```python
from build123d import *

# Parameters (mm, degrees)
SKETCH1_R               = 72.5
SKETCH1_R_2             = 62.5
BOSS_EXTRUDE1_DEPTH     = 10
SKETCH2_W               = 25
SKETCH2_H               = 10
BOSS_EXTRUDE2_DEPTH     = 100
SKETCH3_W               = 145
SKETCH3_H               = 50
BOSS_EXTRUDE3_DEPTH     = 10
CUT_EXTRUDE1_START      = -10
SKETCH4_R               = 62.5
CUT_EXTRUDE1_DEPTH      = 10
SKETCH5_W               = 145
SKETCH5_H               = 12.5
BOSS_EXTRUDE4_DEPTH     = 50
CUT_EXTRUDE2_DEPTH      = 138.318061449
CUT_EXTRUDE2_DEPTH_BACK = 138.318061449
SKETCH6_R               = 1.75
CUT_EXTRUDE3_DEPTH      = 138.318061449
CUT_EXTRUDE3_DEPTH_BACK = 138.318061449
SKETCH7_W               = 2.5
SKETCH7_H               = 7.5
SKETCH8_W               = 145
SKETCH8_H               = 12.5
CUT_EXTRUDE4_DEPTH      = 50
SKETCH9_W               = 145
SKETCH9_H               = 10
CUT_EXTRUDE5_DEPTH      = 87.5
SKETCH11_W              = 12.5
SKETCH11_H              = 10
CUT_EXTRUDE7_DEPTH      = 15
SKETCH13_W              = 12.5
SKETCH13_H              = 10
CUT_EXTRUDE9_DEPTH      = 50
SKETCH14_W              = 12.5
SKETCH14_H              = 10
CUT_EXTRUDE10_DEPTH     = 25


with BuildPart() as part:
    # Sketch1 → Boss-Extrude1 (new body)
    with BuildSketch(Plane(origin=(0, 0, 0), x_dir=(1, 0, 0), z_dir=(0, 1, 0))):
        with Locations(Location((0, 0, 0), (0, 0, 270))):
            Circle(SKETCH1_R)
        with Locations(Location((0, 0, 0), (0, 0, 270))):
            Circle(SKETCH1_R_2, mode=Mode.SUBTRACT)
    extrude(amount=BOSS_EXTRUDE1_DEPTH)

    # Sketch2 → Boss-Extrude2 (add)
    with BuildSketch(Plane.XY):
        with Locations((-60, 5)):
            Rectangle(SKETCH2_W, SKETCH2_H)
        with Locations((60, 5)):
            Rectangle(SKETCH2_W, SKETCH2_H)
    extrude(amount=BOSS_EXTRUDE2_DEPTH)

    # Sketch3 → Boss-Extrude3 (add)
    with BuildSketch(Plane(origin=(0, 10, 0), x_dir=(1, 0, 0), z_dir=(0, 1, 0))):
        with Locations((0, -75)):
            Rectangle(SKETCH3_W, SKETCH3_H)
    extrude(amount=-BOSS_EXTRUDE3_DEPTH)

    # Sketch4 → Cut-Extrude1 (cut)
    with BuildSketch(Plane(origin=(0, 10, 0), x_dir=(1, 0, 0), z_dir=(0, 1, 0)).offset(CUT_EXTRUDE1_START)):
        with Locations(Location((0, 0, 0), (0, 0, 270))):
            Circle(SKETCH4_R)
    extrude(amount=CUT_EXTRUDE1_DEPTH, mode=Mode.SUBTRACT)

    # Sketch5 → Boss-Extrude4 (add)
    with BuildSketch(Plane(origin=(0, 10, 0), x_dir=(1, 0, 0), z_dir=(0, 1, 0))):
        with Locations((0, -93.75)):
            Rectangle(SKETCH5_W, SKETCH5_H)
    extrude(amount=BOSS_EXTRUDE4_DEPTH)

    # Sketch6 → Cut-Extrude2 (cut, two sides: drawn at the far end of the back side and taken through both)
    with BuildSketch(Plane.XZ.offset(-CUT_EXTRUDE2_DEPTH_BACK)):
        with Locations(Location((-50.65, 95, 0), (0, 0, 270))):
            Circle(SKETCH6_R)
        with Locations(Location((-13.15, 95, 0), (0, 0, 270))):
            Circle(SKETCH6_R)
        with Locations(Location((24.35, 95, 0), (0, 0, 270))):
            Circle(SKETCH6_R)
        with Locations(Location((61.85, 95, 0), (0, 0, 270))):
            Circle(SKETCH6_R)
    extrude(amount=CUT_EXTRUDE2_DEPTH + CUT_EXTRUDE2_DEPTH_BACK, mode=Mode.SUBTRACT)

    # Sketch7 → Cut-Extrude3 (cut, two sides: drawn at the far end of the back side and taken through both)
    with BuildSketch(Plane.XZ.offset(-CUT_EXTRUDE3_DEPTH_BACK)):
        with Locations((-13.15, 100)):
            Rectangle(SKETCH7_W, SKETCH7_H)
        with Locations((-50.65, 100)):
            Rectangle(SKETCH7_W, SKETCH7_H)
        with Locations((24.35, 100)):
            Rectangle(SKETCH7_W, SKETCH7_H)
        with Locations((61.85, 100)):
            Rectangle(SKETCH7_W, SKETCH7_H)
    extrude(amount=CUT_EXTRUDE3_DEPTH + CUT_EXTRUDE3_DEPTH_BACK, mode=Mode.SUBTRACT)

    # Sketch8 → Cut-Extrude4 (cut)
    with BuildSketch(Plane(origin=(0, 60, 0), x_dir=(1, 0, 0), z_dir=(0, 1, 0))):
        with Locations((0, -93.75)):
            Rectangle(SKETCH8_W, SKETCH8_H)
    extrude(amount=-CUT_EXTRUDE4_DEPTH, mode=Mode.SUBTRACT)

    # Sketch9 → Cut-Extrude5 (cut, symmetric)
    with BuildSketch(Plane.XY):
        with Locations((0, 5)):
            Rectangle(SKETCH9_W, SKETCH9_H)
    extrude(amount=CUT_EXTRUDE5_DEPTH, both=True, mode=Mode.SUBTRACT)

    # Sketch11 → Cut-Extrude7 (cut)
    with BuildSketch(Plane(origin=(72.5, 0, 0), x_dir=(0, 0, -1), z_dir=(1, 0, 0))):
        with Locations((-93.75, 5)):
            Rectangle(SKETCH11_W, SKETCH11_H)
    extrude(amount=-CUT_EXTRUDE7_DEPTH, mode=Mode.SUBTRACT)

    # Sketch13 → Cut-Extrude9 (cut)
    with BuildSketch(Plane.ZY.offset(72.5)):
        with Locations((93.75, 5)):
            Rectangle(SKETCH13_W, SKETCH13_H)
    extrude(amount=-CUT_EXTRUDE9_DEPTH, mode=Mode.SUBTRACT)

    # Sketch14 → Cut-Extrude10 (cut)
    with BuildSketch(Plane(origin=(57.5, 0, 0), x_dir=(0, 0, -1), z_dir=(1, 0, 0))):
        with Locations((-93.75, 5)):
            Rectangle(SKETCH14_W, SKETCH14_H)
    extrude(amount=-CUT_EXTRUDE10_DEPTH, mode=Mode.SUBTRACT)


solid = part.part
```
Geometry check sheet. Reference: the model listing, model coordinates, mm. A direction names the side the tool comes from. Coordinates: 2 decimals unless noted, no trailing zeros. Order: outer loops, then holes, each group sorted by start corner. A loop starts at its lowest first (then second) coordinate and runs counter-clockwise, first axis right, second up. Notation, with made-up numbers: M 13.25,54 L 51.25,54 A19 ccw 51.25,90 Z; hole C 78.25,-5.75 d6. An arc over 180 degrees is marked long. Answer as a JSON object with one key per item and string values.
Q1. Cross-section at D-D on x = 24.35. Record the cut outline in (y, z), and give its area (3 significant figures).
Results are:
{"outline": "M 0,87.5 L 10,87.5 L 10,93.25 L 0,93.25 Z", "area": "57.5 mm²"}
Q2. Cross-section at C-C on z = 93.75. Record the cut outline in (x, y).
Results are:
{"outline": "M -22.5,0 L -14.37,0 L -14.37,10 L -22.5,10 Z; M -11.93,0 L 23.13,0 L 23.13,10 L -11.93,10 Z; M 25.57,0 L 32.5,0 L 32.5,10 L 25.57,10 Z"}
Q3. Scan lines: line 1 (X direction, y = 6.5, z = 95); line 2 (X direction, y = 8.5, z = 97.5). Record each from-to range of solid material in increasing order.
Results are:
{"line 1": "x = -22.5 to -14.9, -11.4 to 22.6, 26.1 to 32.5", "line 2": "x = -22.5 to -14.4, -11.9 to 23.1, 25.6 to 32.5"}
Q4. Tool access check on faces 4 (the flat face through (32.5, 5, 94)), 5 (the flat face through (23.1, 5, 98)). Record the directions out of +Z, -Z, +X, -X, +Y, -Y that give a thin tool (end or side, any length) a straight path to the whole face; none if there is none.
Results are:
{"face 4": "+Z, -Z, +X, +Y, -Y", "face 5": "+Z, +Y, -Y"}
Q5. Cross-section at A-A on z = 97.25. Record the cut outline in (x, y).
Results are:
{"outline": "M -22.5,0 L -14.4,0 L -14.4,10 L -22.5,10 Z; M -11.9,0 L 23.1,0 L 23.1,10 L -11.9,10 Z; M 25.6,0 L 32.5,0 L 32.5,10 L 25.6,10 Z"}
Q6. Release check for a two-part mould opening along Z. For faces 1 (the flat face through (-14.4, 5, 98)), 2 (the flat face through (5, 5, 87.5)), 3 (the cylindrical face through (-13.21, 5.07, 93.25)) record: released by +Z, released by -Z, zero draft, split by the parting line, or undercut.
Results are:
{"face 1": "zero draft", "face 2": "released by -Z", "face 3": "undercut"}
